Design review of the part shown in the three views and the two pictorial views. Dimensions are in mm from the part's minimum x, y and z. Give positions to 0.01 mm unless a question says otherwise; leave off trailing zeros. Loops run counter-clockwise (first coordinate to the right, second up) from the corner with the lowest first, then second, coordinate; pieces in that order, holes last. Notation, with made-up numbers: (23.25, 29) - (47.25, 29) arc R18 ccw to (47.25, 64) - close; hole circle Ø8 at (61.25, 88.25). An arc over 180 degrees is marked (long way). Answer in a Markdown table with one row per item.
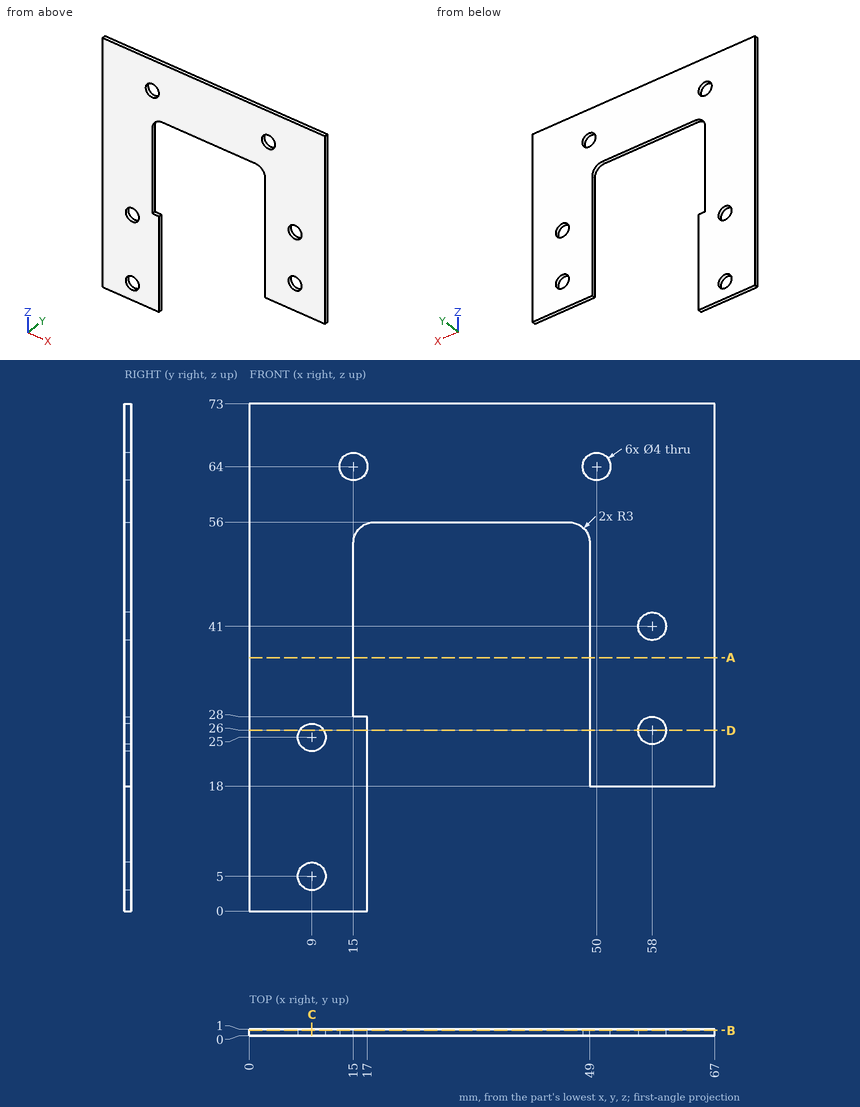
1. We need section A-A, the plane z = 36.5. Give the boundary of the cut face in (x, y).
Values:
| item | result |
|---|---|
| outline | (0, 0) - (15, 0) - (15, 1) - (0, 1) - close; (49, 0) - (67, 0) - (67, 1) - (49, 1) - close |
2. We need section C-C, the plane x = 9. Give the boundary of the cut face in (y, z), and give its area (3 significant figures).
Values:
| item | result |
|---|---|
| outline | (0, 0) - (1, 0) - (1, 3) - (0, 3) - close; (0, 7) - (1, 7) - (1, 23) - (0, 23) - close; (0, 27) - (1, 27) - (1, 73) - (0, 73) - close |
| area | 65.0 mm^2 |
3. We need section D-D, the plane z = 26. Give the boundary of the cut face in (x, y), and give its area (3 significant figures).
Values:
| item | result |
|---|---|
| outline | (0, 0) - (7.27, 0) - (7.27, 1) - (0, 1) - close; (10.73, 0) - (17, 0) - (17, 1) - (10.73, 1) - close; (49, 0) - (56, 0) - (56, 1) - (49, 1) - close; (60, 0) - (67, 0) - (67, 1) - (60, 1) - close |
| area | 27.5 mm^2 |
4. Wall thickness on line 1 (Z direction, x = 58, y = 0.35); line 2 (Z direction, x = 9, y = 0.7); line 3 (X direction, y = 0.2, z = 64): over which ranges is each line inside the solid? List them lowest first. Write a range as [from, to].
Values:
| item | result |
|---|---|
| line 1 | z = [18, 24], [28, 39], [43, 73] |
| line 2 | z = [0, 3], [7, 23], [27, 73] |
| line 3 | x = [0, 13], [17, 48], [52, 67] |
5. We need section B-B, the plane y = 0.8. Give the boundary of the cut face in (x, z), and give its area (3 significant figures).
Values:
| item | result |
|---|---|
| outline | (0, 0) - (17, 0) - (17, 28) - (15, 28) - (15, 53) arc R3 cw to (18, 56) - (46, 56) arc R3 cw to (49, 53) - (49, 18) - (67, 18) - (67, 73) - (0, 73) - close; hole circle Ø4 at (9, 5); hole circle Ø4 at (9, 25); hole circle Ø4 at (15, 64); hole circle Ø4 at (50, 64); hole circle Ø4 at (58, 26); hole circle Ø4 at (58, 41) |
| area | 2,650 mm^2 |
6. Clearance check with a flat-ended pin moving along its axis: pin 1 (0.5 mm diameter, centred on y = 0.5, z = 13.5, fed in from +X). State where the tip first meets the part, or that it passes through.
Values:
| item | result |
|---|---|
| pin 1 | stops at x = 17 |
